```python
from build123d import *

# Parameters (mm, degrees)
FILLET1_R               = 0.5
CUT_EXTRUDE1_DEPTH      = 78.97595784
CIRPATTERN1_COUNT       = 3
CUT_EXTRUDE2_DEPTH      = 78.975957833
CUT_EXTRUDE2_DEPTH_BACK = 78.975957833
SKETCH3_R               = 3
BOSS_EXTRUDE1_DEPTH     = 1.5
CUT_EXTRUDE3_DEPTH      = 78.839578622
CUT_EXTRUDE3_DEPTH_BACK = 78.839578622
SKETCH6_R               = 2.75
SKETCH7_R               = 9.5
SKETCH7_R_2             = 3
BOSS_EXTRUDE2_DEPTH     = 5
CUT_EXTRUDE5_DEPTH      = 78.942286341
CUT_EXTRUDE5_DEPTH_BACK = 78.942286341
SKETCH9_R               = 5.5


# Read off the part's stored shape, not the designer's step: Split1, Split2
with BuildPart() as part:
    # Sketch1 → Revolve1 (revolve)
    with BuildSketch(Plane(origin=(0, 0, 0), x_dir=(0, 0, -1), z_dir=(1, 0, 0)), mode=Mode.PRIVATE) as revolve1_sk:
        Polygon((-4, 55), (4, 55), (4, 50), (1.5, 50), (1.5, 0), (-1.5, 0), (-1.5, 50), (-4, 50), align=None)
    revolve(revolve1_sk.sketch.rotate(Axis((0, 0, 1.5), (0, 0, -1)), 90), axis=Axis((0, 0, 1.5), (0, 0, -1)))

    # Fillet1
    fillet1_edges = [part.edges().sort_by_distance(p)[0] for p in [
        (-50, 0, -1.5),
        (-50, 0, -4),
        (-55, 0, -4),
        (-55, 0, 4),
        (-50, 0, 4),
        (-50, 0, 1.5),
    ]]
    fillet(fillet1_edges, radius=FILLET1_R)

    # Sketch2 → Cut-Extrude1 (cut, symmetric)
    with BuildSketch(Plane(origin=(0, 0, -1.5), x_dir=(-1, 0, 0), z_dir=(0, 0, -1))):
        with BuildLine():
            Line((10.633924434, -3.830098058), (41.516200464, -21.659988437))
            ThreePointArc((41.516200464, -21.659988437), (43.528240329, -21.875953118), (45.040998361, -20.531889019))
            ThreePointArc((45.040998361, -20.531889019), (42.868257487, 24.75), (4.739361702, 49.272593302))
            ThreePointArc((4.739361702, 49.272593302), (2.818989033, 48.634538466), (2, 46.784078488))
            Line((2, 46.784078488), (2, 11.124297731))
            ThreePointArc((2, 11.124297731), (2.427109506, 9.726755245), (3.5625, 8.806735703))
            ThreePointArc((3.5625, 8.806735703), (8.227241336, 4.75), (9.408106844, -1.318152351))
            ThreePointArc((9.408106844, -1.318152351), (9.637171891, -2.761439132), (10.633924434, -3.830098058))
        make_face()
    cut_extrude1 = extrude(amount=CUT_EXTRUDE1_DEPTH, both=True, mode=Mode.SUBTRACT)

    # CirPattern1: Cut-Extrude1 ×3 about axis
    cirpattern1_axis = Axis((0, 0, 0), (0, 0, 1))
    for i in range(1, CIRPATTERN1_COUNT):
        add(cut_extrude1.rotate(cirpattern1_axis, i * 360 / CIRPATTERN1_COUNT), mode=Mode.SUBTRACT)

    # Sketch3 → Cut-Extrude2 (cut, two sides: drawn at the far end of the back side and taken through both)
    with BuildSketch(Plane.XY.offset(1.5).offset(-CUT_EXTRUDE2_DEPTH_BACK)):
        Circle(SKETCH3_R)
    extrude(amount=CUT_EXTRUDE2_DEPTH + CUT_EXTRUDE2_DEPTH_BACK, mode=Mode.SUBTRACT)

    # Sketch4 → Boss-Extrude1 (add, symmetric)
    with BuildSketch(Plane.XY):
        with BuildLine():
            Line((-2, 46.784078488), (-2, 34.441980199))
            ThreePointArc((-2, 34.441980199), (-29.877876431, 17.25), (-30.827629809, -15.488939292))
            Line((-30.827629809, -15.488939292), (-41.516200464, -21.659988437))
            ThreePointArc((-41.516200464, -21.659988437), (-43.528240329, -21.875953118), (-45.040998361, -20.531889019))
            ThreePointArc((-45.040998361, -20.531889019), (-42.868257487, 24.75), (-4.739361702, 49.272593302))
            ThreePointArc((-4.739361702, 49.272593302), (-2.818989033, 48.634538466), (-2, 46.784078488))
        make_face()
        with BuildLine():
            Line((2, 34.441980199), (2, 46.784078488))
            ThreePointArc((2, 46.784078488), (2.818989033, 48.634538466), (4.739361702, 49.272593302))
            ThreePointArc((4.739361702, 49.272593302), (42.868257487, 24.75), (45.040998361, -20.531889019))
            ThreePointArc((45.040998361, -20.531889019), (43.528240329, -21.875953118), (41.516200464, -21.659988437))
            Line((41.516200464, -21.659988437), (30.827629809, -15.488939292))
            ThreePointArc((30.827629809, -15.488939292), (29.877876431, 17.25), (2, 34.441980199))
        make_face()
        with BuildLine():
            Line((28.827629809, -18.953040907), (39.516200464, -25.124090052))
            ThreePointArc((39.516200464, -25.124090052), (40.709251296, -26.758585348), (40.301636658, -28.740704283))
            ThreePointArc((40.301636658, -28.740704283), (0, -49.5), (-40.301636658, -28.740704283))
            ThreePointArc((-40.301636658, -28.740704283), (-40.709251296, -26.758585348), (-39.516200464, -25.124090052))
            Line((-39.516200464, -25.124090052), (-28.827629809, -18.953040907))
            ThreePointArc((-28.827629809, -18.953040907), (0, -34.5), (28.827629809, -18.953040907))
        make_face()
    extrude(amount=BOSS_EXTRUDE1_DEPTH, both=True)


with BuildPart() as body_2:
    # Split1: the piece on the far side of the plane
    add(part.part)
    split(bisect_by=Plane.XY.offset(1.5), keep=Keep.BOTTOM)


with BuildPart() as part_1:
    add(part.part)

    # Split1
    split(bisect_by=Plane.XY.offset(1.5), keep=Keep.TOP)


with BuildPart() as body_3:
    # Split2: the piece on the far side of the plane
    add(body_2.part)
    split(bisect_by=Plane.XY.offset(-1.5), keep=Keep.BOTTOM)


with BuildPart() as body_2_1:
    add(body_2.part)

    # Split2
    split(bisect_by=Plane.XY.offset(-1.5), keep=Keep.TOP)

    # Sketch6 → Cut-Extrude3 (cut, two sides: drawn at the far end of the back side and taken through both)
    with BuildSketch(Plane(origin=(0, 0, -1.5), x_dir=(-1, 0, 0), z_dir=(0, 0, -1)).offset(-CUT_EXTRUDE3_DEPTH_BACK)):
        with Locations((-44.75, 0)):
            Circle(SKETCH6_R)
        with Locations((-41.34360908, 17.125083598)):
            Circle(SKETCH6_R)
        with Locations((-31.643028458, 31.643028458)):
            Circle(SKETCH6_R)
        with Locations((-17.125083598, 41.34360908)):
            Circle(SKETCH6_R)
        with Locations((0, 44.75)):
            Circle(SKETCH6_R)
        with Locations((17.125083598, 41.34360908)):
            Circle(SKETCH6_R)
        with Locations((31.643028458, 31.643028458)):
            Circle(SKETCH6_R)
        with Locations((41.34360908, 17.125083598)):
            Circle(SKETCH6_R)
        with Locations((44.75, 0)):
            Circle(SKETCH6_R)
        with Locations((41.34360908, -17.125083598)):
            Circle(SKETCH6_R)
        with Locations((31.643028458, -31.643028458)):
            Circle(SKETCH6_R)
        with Locations((17.125083598, -41.34360908)):
            Circle(SKETCH6_R)
        with Locations((0, -44.75)):
            Circle(SKETCH6_R)
        with Locations((-17.125083598, -41.34360908)):
            Circle(SKETCH6_R)
        with Locations((-31.643028458, -31.643028458)):
            Circle(SKETCH6_R)
        with Locations((-41.34360908, -17.125083598)):
            Circle(SKETCH6_R)
    extrude(amount=CUT_EXTRUDE3_DEPTH + CUT_EXTRUDE3_DEPTH_BACK, mode=Mode.SUBTRACT)

    # Sketch7 → Boss-Extrude2 (add)
    with BuildSketch(Plane.XY.offset(1.5)):
        with Locations(Location((0, 0, 0), (0, 0, 180))):
            Circle(SKETCH7_R)
        Circle(SKETCH7_R_2, mode=Mode.SUBTRACT)
    extrude(amount=BOSS_EXTRUDE2_DEPTH)

    # Sketch9 → Cut-Extrude5 (cut, two sides: drawn at the far end of the back side and taken through both)
    with BuildSketch(Plane.XY.offset(1.5).offset(-CUT_EXTRUDE5_DEPTH_BACK)):
        Circle(SKETCH9_R)
    extrude(amount=CUT_EXTRUDE5_DEPTH + CUT_EXTRUDE5_DEPTH_BACK, mode=Mode.SUBTRACT)


solid = body_2_1.part
```
CAD build for the part. Positions are in the model's coordinates, mm. Round coordinates to 2 decimals unless told otherwise and drop trailing zeros. Write each loop counter-clockwise with the first axis right and the second up, starting at its lowest first coordinate (ties: lowest second). Pieces come first, ordered by that corner, then holes. Notation, with made-up numbers: (59.5, 50) - (116.5, 50) arc R25 cw to (116.5, 63) - close; hole circle Ø4 at (67.25, -35.75). An arc over 180 degrees is marked (long way). Return JSON: item names as keys, results as strings. Group by question number.
Item 1: Mould opens along X. For faces 1 (the face through (-2, 23, 0)), 2 (the face through (1, 13, 1.5)) say: +X half, -X half, draft (parallel to the pull), parting line (faces both ways), or undercut.
Item 2: Band-saw the part on A-A on x = 0. List the corners of the cut face in (y, z), plus the area to 3 significant figures.
Item 3: Band-saw the part on C-C on y = -33. List the corners of the cut face in (x, z).
Item 4: Flat gauge pins, fed straight in: pin 1 Ø3.5 at (x, y) = (17.13, -41.34) entering from -Z; pin 2 Ø1.5 at (x, z) = (-6, 0.5) entering from -Y; pin 3 Ø7 at (x, y) = (0, -44.75) entering from -Z; pin 4 Ø0.9 at (y, z) = (19, 0.5) entering from +X. Where does each tip first touch, or does it go through?
Item 5: Probe probe 1 along X at (y, z) = (23, -0.5); probe 2 along Y at (x, z) = (43.5, 0.5); probe 3 along X at (y, z) = (22.5, -0.5). List the from-to ranges inside material, lowest first.
Item 6: Band-saw the part on D-D on z = 2.75. List the corners of the cut face in (x, y), plus the area to 3 significant figures.
Item 7: Band-saw the part on B-B on y = 0. List the corners of the cut face in (x, z), plus the area to 3 significant figures.
Resolved:
{
 "1": {"face 1": "undercut", "face 2": "draft"},
 "2": {"outline": "(-55, -1.5) - (-47.5, -1.5) - (-47.5, 1.5) - (-55, 1.5) - close; (-42, -1.5) - (-34.5, -1.5) - (-34.5, 1.5) - (-42, 1.5) - close; (-9.5, -1.5) - (-5.5, -1.5) - (-5.5, 6.5) - (-9.5, 6.5) - close; (5.5, -1.5) - (42, -1.5) - (42, 1.5) - (9.5, 1.5) - (9.5, 6.5) - (5.5, 6.5) - close; (47.5, -1.5) - (55, -1.5) - (55, 1.5) - (47.5, 1.5) - close", "area": "229 mm²"},
 "3": {"outline": "(-44, -1.5) - (-34.03, -1.5) - (-34.03, 1.5) - (-44, 1.5) - close; (-29.25, -1.5) - (-10.06, -1.5) - (-10.06, 1.5) - (-29.25, 1.5) - close; (10.06, -1.5) - (29.25, -1.5) - (29.25, 1.5) - (10.06, 1.5) - close; (34.03, -1.5) - (44, -1.5) - (44, 1.5) - (34.03, 1.5) - close"},
 "4": {"pin 1": "passes through", "pin 2": "stops at y = -54.75", "pin 3": "stops at z = -1.5", "pin 4": "stops at x = 51.78"},
 "5": {"probe 1": "x = -49.96 to -25.71, -2 to 2, 25.71 to 49.96", "probe 2": "y = -33.66 to -18.83, -15.42 to -2.45, 2.45 to 15.42, 18.83 to 33.66", "probe 3": "x = -50.19 to -26.15, -2 to 2, 26.15 to 50.19"},
 "6": {"outline": "circle Ø19 at (0, 0); hole circle Ø11 at (0, 0)", "area": "188 mm²"},
 "7": {"outline": "(-55, -1.5) - (-47.5, -1.5) - (-47.5, 1.5) - (-55, 1.5) - close; (-42, -1.5) - (-34.5, -1.5) - (-34.5, 1.5) - (-42, 1.5) - close; (-9.5, -1.5) - (-5.5, -1.5) - (-5.5, 6.5) - (-9.5, 6.5) - close; (5.5, -1.5) - (9.5, -1.5) - (9.5, 6.5) - (5.5, 6.5) - close; (34.5, -1.5) - (42, -1.5) - (42, 1.5) - (34.5, 1.5) - close; (47.5, -1.5) - (55, -1.5) - (55, 1.5) - (47.5, 1.5) - close", "area": "154 mm²"}
}
